```python
from build123d import *

# Parameters (mm, degrees)
PAD_DEPTH       = 1.9
SKETCH001_R     = 4.45
POCKET_DEPTH    = 0.7
SKETCH002_R     = 3.45
PAD001_DEPTH    = 0.8
SKETCH003_R     = 3
POCKET001_DEPTH = 0.8
SKETCH004_R     = 4.9
PAD002_DEPTH    = 1
SKETCH005_R     = 4.185
PAD003_DEPTH    = 2.9
SKETCH006_R     = 2.95
POCKET002_DEPTH = 3.9
SKETCH007_R     = 1.45
POCKET003_DEPTH = 2.001
CHAMFER_SIZE    = 0.3
CHAMFER001_SIZE = 0.3
CHAMFER002_SIZE = 0.3
SKETCH008_R     = 0.8
POCKET004_DEPTH = 88.048918
FILLET_R        = 0.1
CHAMFER003_SIZE = 0.1


with BuildPart() as horn_top_left_quarter:
    # Sketch → Pad (new body)
    with BuildSketch(Plane.XY):
        with BuildLine():
            ThreePointArc((0, 6.45), (-2.239283, 6.048811), (-4.2, 4.895151))
            ThreePointArc((-5.52408, 4.1), (-4.751834, 4.314062), (-4.2, 4.895151))
            Line((-17.197947, 2.425167), (-5.52408, 4.1))
            ThreePointArc((-17.197947, 2.425167), (-18.701347, 1.604685), (-19.3, 0))
            Line((-19.3, 0), (0, 0))
            Line((0, 6.45), (0, 0))
        make_face()
    extrude(amount=PAD_DEPTH)


with BuildPart() as horn_top_half:
    # Part__Mirroring: instance of horn-top-left-quarter
    add(horn_top_left_quarter.part.mirror(Plane(origin=(0, 0, 0), x_dir=(0, -1, 0), z_dir=(1, 0, 0))))

    # Fusion: union horn-top-left-quarter
    add(horn_top_left_quarter.part)


with BuildPart() as horn_final001:
    # Part__Mirroring001: instance of horn-top-half
    add(horn_top_half.part.mirror(Plane(origin=(0, 0, 0), x_dir=(1, 0, 0), z_dir=(0, 1, 0))))

    # Fusion001: union horn-top-half
    add(horn_top_half.part)

    # Sketch001 → Pocket (cut)
    with BuildSketch(Plane.XY.offset(1.9)):
        with Locations((0.021849, -0.030682)):
            Circle(SKETCH001_R)
    extrude(amount=-POCKET_DEPTH, mode=Mode.SUBTRACT)

    # Sketch002 → Pad001 (new body)
    with BuildSketch(Plane.XY.offset(1.2)):
        Circle(SKETCH002_R)
    extrude(amount=PAD001_DEPTH)

    # Sketch003 → Pocket001 (cut)
    with BuildSketch(Plane.XY.offset(2)):
        Circle(SKETCH003_R)
    extrude(amount=-POCKET001_DEPTH, mode=Mode.SUBTRACT)

    # Sketch004 → Pad002 (new body)
    with BuildSketch(Plane(origin=(0, 0, 0), x_dir=(1, 0, 0), z_dir=(0, 0, -1))):
        Circle(SKETCH004_R)
    extrude(amount=PAD002_DEPTH)

    # Sketch005 → Pad003 (new body)
    with BuildSketch(Plane(origin=(0, 0, -1), x_dir=(1, 0, 0), z_dir=(0, 0, -1))):
        Circle(SKETCH005_R)
    extrude(amount=PAD003_DEPTH)

    # Sketch006 → Pocket002 (cut)
    with BuildSketch(Plane(origin=(0, 0, -3.9), x_dir=(1, 0, 0), z_dir=(0, 0, -1))):
        Circle(SKETCH006_R)
    extrude(amount=-POCKET002_DEPTH, mode=Mode.SUBTRACT)

    # Sketch007 → Pocket003 (cut, through all)
    with BuildSketch(Plane(origin=(0, 0, 0), x_dir=(1, 0, 0), z_dir=(0, 0, -1))):
        Circle(SKETCH007_R)
    extrude(amount=-POCKET003_DEPTH, mode=Mode.SUBTRACT)

    # Chamfer
    chamfer_edges = [horn_final001.edges().sort_by_distance(p)[0] for p in [
        (-4.9, 0, 0),
    ]]
    chamfer(chamfer_edges, length=CHAMFER_SIZE)

    # Chamfer001
    chamfer001_edges = [horn_final001.edges().sort_by_distance(p)[0] for p in [
        (-4.185, 0, -1),
    ]]
    chamfer(chamfer001_edges, length=CHAMFER001_SIZE)

    # Chamfer002
    chamfer002_edges = [horn_final001.edges().sort_by_distance(p)[0] for p in [
        (-4.9, 0, -1),
    ]]
    chamfer(chamfer002_edges, length=CHAMFER002_SIZE)

    # Sketch008 → Pocket004 (cut, through all)
    with BuildSketch(Plane.XY.offset(1.9)):
        with Locations((-16.15, 0)):
            Circle(SKETCH008_R)
        with Locations((-13.03, 0)):
            Circle(SKETCH008_R)
        with Locations((-10.035, 0)):
            Circle(SKETCH008_R)
        with Locations((-7.51, 0)):
            Circle(SKETCH008_R)
    pocket004 = extrude(amount=-POCKET004_DEPTH, mode=Mode.SUBTRACT)

    # Mirrored: Pocket004 across Sketch008 V_Axis
    add(pocket004.mirror(Plane(origin=(0, 0, 1.9), x_dir=(0, 0, 1), z_dir=(1, 0, 0))), mode=Mode.SUBTRACT)

    # Fillet
    fillet_edges = [horn_final001.edges().sort_by_distance(p)[0] for p in [
        (-4.185, 0, -3.9),
    ]]
    fillet(fillet_edges, radius=FILLET_R)

    # Chamfer003
    chamfer003_edges = [horn_final001.edges().sort_by_distance(p)[0] for p in [
        (-2.95, 0, -3.9),
    ]]
    chamfer(chamfer003_edges, length=CHAMFER003_SIZE)


solid = horn_final001.part
```
Model file for the job. Use its own axes, mm. A direction names the side the tool comes from. Give positions to 0.01 mm unless a question says otherwise; leave off trailing zeros. Write each loop counter-clockwise with the first axis right and the second up, starting at its lowest first coordinate (ties: lowest second). Pieces come first, ordered by that corner, then holes. Notation, with made-up numbers: (88.25, 74.5) -> (96.25, 74.5) arc R26 ccw to (96.25, 89.5) -> close; hole circle Ø10 at (81.25, 17). An arc over 180 degrees is marked (long way). Use CSV: the item, a comma, the result in double quotes. Start each with the question number.
1) Tool access for faces 4 (the flat face through (-11.44, 3.25, 0.94)), 5 (the flat face through (2, -3, 1.2)), 6 (the cylindrical face through (-2.947, -0.13, -1.927)): list every direction of +Z, -Z, +X, -X, +Y, -Y with a clear straight run to the whole face (end or side of a thin tool).
2) Pin check, flat tips, straight feed: P1, Ø1, axis at x = 2, y = 1.5, coming from the -Z side; P2, Ø2.5, axis at x = 7.51, y = 0, coming from the +Z side; P3, Ø3, axis at x = 14, y = -2.5, coming from the -Z side. Stop position of each tip, or through.
3) Drill centre lines: L1, parallel to Z at x = -2.5, y = -5; L2, parallel to X at y = 1.75, z = -1.35; L3, parallel to Y at x = -13.03, z = 1.4. Where is each one in solid material? Low to high.
4) Two-plate mould, pull along Y, no slides. Class faces 1 (the flat face through (-5, -3, 0)), 2 (the cylindrical face through (-4.76, -4.31, 0.94)), 3 (the cylindrical face through (9.27, 0.24, 0.96)): released by +Y, released by -Y, zero draft, split by the parting line, or undercut.
5) Cut at B-B on x = -7.51. List the corners of the cut face in (y, z).
6) Cut at A-A on x = -13.03. List the corners of the cut face in (y, z).
Final values:
1,face 4,"+Z, -Z, -X, +Y"
1,face 5,"+Z"
1,face 6,"-Z"
2,P1,"stops at z = -3.85"
2,P2,"stops at z = 1.9"
2,P3,"stops at z = 0"
3,L1,"z = 0 to 1.9"
3,L2,"x = -3.8 to -2.37, 2.37 to 3.8"
3,L3,"y = -3.02 to -0.8, 0.8 to 3.02"
4,face 1,"zero draft"
4,face 2,"released by -Y"
4,face 3,"undercut"
5,outline,"(-3.82, 0) -> (-0.8, 0) -> (-0.8, 1.9) -> (-3.82, 1.9) -> close; (0.8, 0) -> (3.82, 0) -> (3.82, 1.9) -> (0.8, 1.9) -> close"
6,outline,"(-3.02, 0) -> (-0.8, 0) -> (-0.8, 1.9) -> (-3.02, 1.9) -> close; (0.8, 0) -> (3.02, 0) -> (3.02, 1.9) -> (0.8, 1.9) -> close"
